from build123d import *

# Parameters (mm, degrees)
SKETCH1_R           = 12.7
BOSS_EXTRUDE1_DEPTH = 5.9182
SKETCH3_R           = 11.1252
BOSS_EXTRUDE2_DEPTH = 1.778
SKETCH4_R           = 7.874
BOSS_EXTRUDE3_DEPTH = 14.859


with BuildPart() as part:
    # Sketch1 → Boss-Extrude1 (new body)
    with BuildSketch(Plane(origin=(0, 0, 0), x_dir=(1, 0, 0), z_dir=(0, 1, 0))):
        with Locations(Location((0, 0, 0), (0, 0, 270))):
            Circle(SKETCH1_R)
    extrude(amount=BOSS_EXTRUDE1_DEPTH)

    # Sketch3 → Boss-Extrude2 (add)
    with BuildSketch(Plane(origin=(0, 5.9182, 0), x_dir=(1, 0, 0), z_dir=(0, 1, 0))):
        with Locations(Location((0, 0, 0), (0, 0, 270))):
            Circle(SKETCH3_R)
    extrude(amount=BOSS_EXTRUDE2_DEPTH)

    # Sketch4 → Boss-Extrude3 (add)
    with BuildSketch(Plane(origin=(0, 7.6962, 0), x_dir=(1, 0, 0), z_dir=(0, 1, 0))):
        with Locations(Location((0, 0, 0), (0, 0, 270))):
            Circle(SKETCH4_R)
    extrude(amount=BOSS_EXTRUDE3_DEPTH)

    # Chamfer2: read off the stored shape, not the designer's step
    # Chamfer2 outline → Chamfer2 (revolve)
    with BuildSketch(Plane.XY):
        Polygon((9.652, 7.6962), (7.874, 9.4742), (7.874, 7.6962), align=None)
    revolve(axis=Axis((0, 0, 0), (0, 1, 0)))


solid = part.part
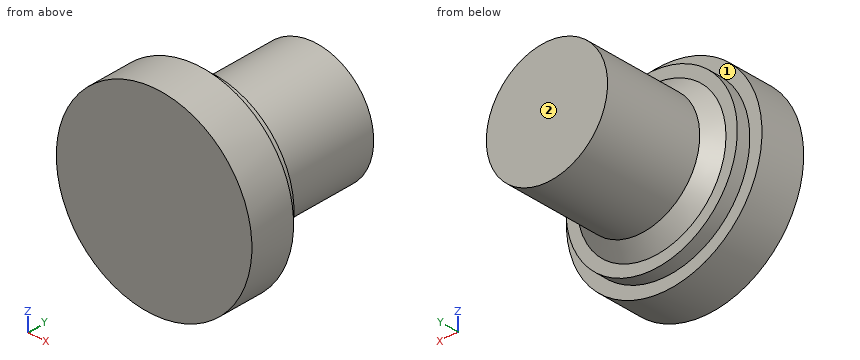
Design review of the part built by this model. Coordinates are the model's own, in mm. Face numbers are marked on the shaded views. A direction names the side the tool comes from. Coordinates: 2 decimals unless noted, no trailing zeros. Loops run counter-clockwise (first coordinate to the right, second up) from the corner with the lowest first, then second, coordinate; pieces in that order, holes last. Notation, with made-up numbers: M 37.25,11 L 85.25,11 A30 cw 85.25,45 Z; hole C 46.5,-22.5 d9. An arc over 180 degrees is marked long. Use one line per item in the form item = value.
(1) For line 1 along Y through (x, z) = (-4, -10.5); line 2 along Y through (x, z) = (10.5, -2.75); line 3 along X through (y, z) = (16.75, -3), list the stretches that pass through material, from the lowest coordinate up. Write a range as from..to.
Return value:
line_1 = 0..5.92
line_2 = 0..7.7
line_3 = -7.28..7.28
(2) Clearance check with flat-ended pins moving along their axes: P1, Ø2, axis at x = -6, y = 18.5, coming from the +Z side; P2, Ø5, axis at x = 9.5, y = 9.5, coming from the -Z side; P3, Ø8, axis at y = 16.5, z = -1, coming from the +X side. State where each tip first meets the part, or that it passes through.
Return value:
P1 = 6.08
P2 = -7.96
P3 = 7.87
(3) Consider section A-A (z = 0). Write out the cut boundary in (x, y).
Return value:
outline = M -12.7,0 L 12.7,0 L 12.7,5.92 L 11.13,5.92 L 11.13,7.7 L 9.65,7.7 L 7.87,9.47 L 7.87,22.56 L -7.87,22.56 L -7.87,9.47 L -9.65,7.7 L -11.13,7.7 L -11.13,5.92 L -12.7,5.92 Z
(4) Consider section B-B (x = 0). Write out the cut boundary in (y, z), and give its area (3 significant figures).
Return value:
outline = M 0,-12.7 L 5.92,-12.7 L 5.92,-11.13 L 7.7,-11.13 L 7.7,-9.65 L 9.47,-7.87 L 22.56,-7.87 L 22.56,7.87 L 9.47,7.87 L 7.7,9.65 L 7.7,11.13 L 5.92,11.13 L 5.92,12.7 L 0,12.7 Z
area = 427 mm2
(5) Consider section D-D (y = 3). Write out the cut boundary in (x, z).
Return value:
outline = C 0,0 d25.4
(6) For the marked faces 1 and 2, list the 3-axis set-ups (+Z, -Z, +X, -X, +Y, -Y) from which the entire face can be reached by the end or side of a thin tool; tool diameter is ignored.
Return value:
face_1 = +Y
face_2 = +Z, -Z, +X, -X, +Y
(7) Consider section C-C (y = 16). Write out the cut boundary in (x, z).
Return value:
outline = C 0,0 d15.75
